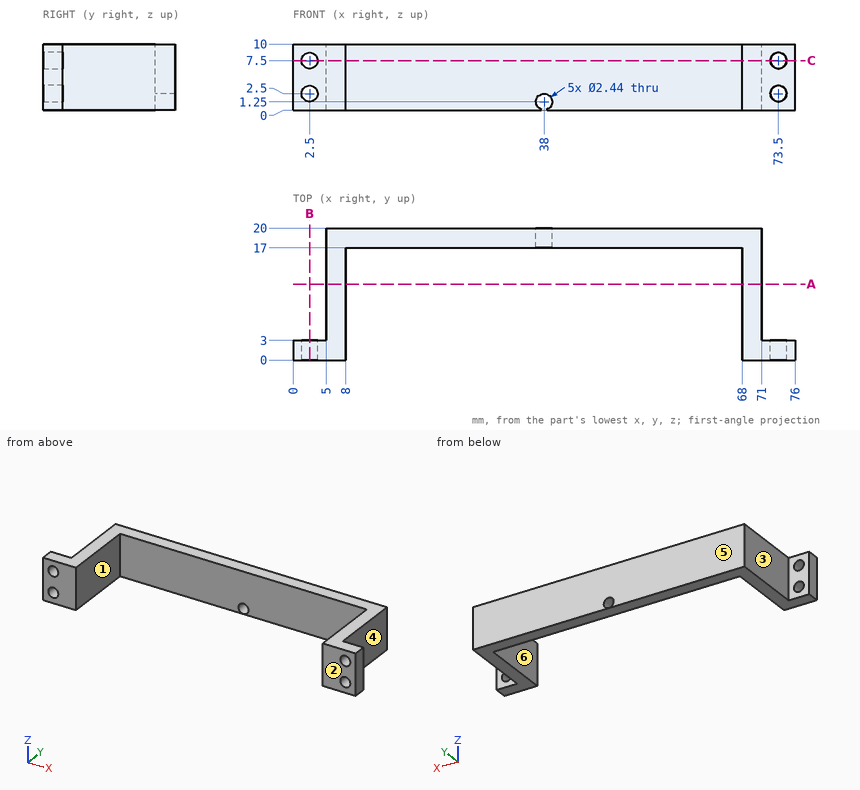
Input: dimensioned drawing with shaded views. Units: mm. Origin: part minimum x, y, z. A direction names the side the tool comes from. Coordinates: 2 decimals unless noted, no trailing zeros. Loops run counter-clockwise (first coordinate to the right, second up) from the corner with the lowest first, then second, coordinate; pieces in that order, holes last. Notation, with made-up numbers: M 85,-18 L 135,-18 A21 cw 135,16 Z; hole C -35,-15.75 d8. An arc over 180 degrees is marked long. One line per item, written item: value. Start each with the question number.
1) Cut plane C-C (z = 7.5). Return loops of the section in (x, y).
2) Cut plane B-B (x = 2.5). Return loops of the section in (y, z).
3) Cut plane A-A (y = 11.5). Return loops of the section in (x, z).
4) Pin query (flat end, axial travel): P1, Ø6, axis at x = 49.5, z = 7.5, coming from the -Y side; P2, Ø6, axis at x = 49, y = 13, coming from the -Z side; P3, Ø3, axis at x = 73.5, z = 7.5, coming from the +Y side; P4, Ø5, axis at y = 12, z = 7, coming from the -X side. Return the tip coordinate at first contact, or that it passes through.
5) Draft query along X for the marked faces 4, 5 and 6. Return one class per face: released by +X, released by -X, zero draft, split by the parting line, or undercut.
6) Reachability of the marked faces 1, 2 and 3 from +Z, -Z, +X, -X, +Y, -Y: full face, straight path, thin tool, end or side. Return the list, or none.
7) Material intervals for L1, parallel to X at y = 2.05, z = 7.5; L2, parallel to X at y = 5, z = 8.5; L3, parallel to X at y = 2.75, z = 1.75, sorted ascending. Write a range as from..to.
Evaluation:
1. outline: M 0,0 L 1.28,0 L 1.28,3 L 0,3 Z; M 3.72,0 L 8,0 L 8,17 L 68,17 L 68,0 L 72.28,0 L 72.28,3 L 71,3 L 71,20 L 5,20 L 5,3 L 3.72,3 Z; M 74.72,0 L 76,0 L 76,3 L 74.72,3 Z
2. outline: M 0,0 L 3,0 L 3,1.28 L 0,1.28 Z; M 0,3.72 L 3,3.72 L 3,6.28 L 0,6.28 Z; M 0,8.72 L 3,8.72 L 3,10 L 0,10 Z
3. outline: M 5,0 L 8,0 L 8,10 L 5,10 Z; M 68,0 L 71,0 L 71,10 L 68,10 Z
4. P1: y = 17
4. P2: through
4. P3: y = 3
4. P4: x = 5
5. face 4: released by +X
5. face 5: zero draft
5. face 6: undercut
6. face 1: +Z, -Z, -Y
6. face 2: +Z, -Z, +X, -X, -Y
6. face 3: +Z, -Z, -X, +Y
7. L1: 0..1.28, 3.72..8, 68..72.28, 74.72..76
7. L2: 5..8, 68..71
7. L3: 0..1.54, 3.46..8, 68..72.54, 74.46..76
